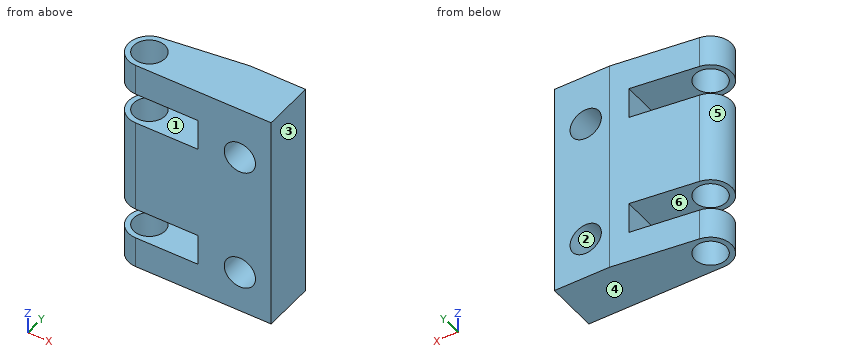
```python
from build123d import *

# Parameters (mm, degrees)
SKETCH_1_R          = 1.5
EXTRUDE_1_DEPTH     = 21
SKETCH_3_W          = 8
SKETCH_3_H          = 3
CUT_EXTRUDE_1_DEPTH = 6
SKETCH_4_R          = 1.5
CUT_EXTRUDE_2_DEPTH = 21


with BuildPart() as part:
    # 草图1 → 凸台-拉伸1 (new body)
    with BuildSketch(Plane.XY):
        with BuildLine():
            Line((-1.936190112, 5), (3.350194549, 5))
            Line((3.350194549, 5), (3.350194549, 0))
            Line((3.350194549, 0), (0, 0))
            Line((0, 0), (-9.649805451, 0))
            ThreePointArc((-9.649805451, 0), (-11.645783707, 1.873229335), (-9.902836943, 3.983929198))
            Line((-9.902836943, 3.983929198), (-1.936190112, 5))
        make_face()
        with Locations((-9.649805451, 2)):
            Circle(SKETCH_1_R, mode=Mode.SUBTRACT)
    extrude(amount=EXTRUDE_1_DEPTH)

    # 草图3 → 切除-拉伸1 (cut, through all)
    with BuildSketch(Plane(origin=(0, 0, 0), x_dir=(1, 0, 0), z_dir=(0, 1, 0))):
        with Locations((-7.649805451, -4.5)):
            Rectangle(SKETCH_3_W, SKETCH_3_H)
        with Locations((-7.649805451, -16.5)):
            Rectangle(SKETCH_3_W, SKETCH_3_H)
    extrude(amount=CUT_EXTRUDE_1_DEPTH, mode=Mode.SUBTRACT)

    # 草图4 → 切除-拉伸2 (cut)
    with BuildSketch(Plane(origin=(0, 5, 0), x_dir=(1, 0, 0), z_dir=(0, 1, 0))):
        with Locations((0.350194549, -4)):
            Circle(SKETCH_4_R)
        with Locations((0.350194549, -16)):
            Circle(SKETCH_4_R)
    extrude(amount=-CUT_EXTRUDE_2_DEPTH, mode=Mode.SUBTRACT)


solid = part.part
```
Input: part model. Units: mm. Frame: model coordinates. Face numbers are marked on the shaded views. A direction names the side the tool comes from. Give positions to 0.01 mm unless a question says otherwise; leave off trailing zeros. Order: outer loops, then holes, each group sorted by start corner. A loop starts at its lowest first (then second) coordinate and runs counter-clockwise, first axis right, second up.
1. Draft query along Z for the marked faces 1, 2, 3 and 4. Return one class per face: released by +Z, released by -Z, zero draft, split by the parting line, or undercut.
Computed:
face 1: undercut
face 2: undercut
face 3: zero draft
face 4: released by -Z
2. Cut plane A-A (y = 2). Return loops of the section in (x, z).
Computed:
outline: (-11.65, 0) - (-11.15, 0) - (-11.15, 3) - (-11.65, 3) - close; (-11.65, 6) - (-11.15, 6) - (-11.15, 15) - (-11.65, 15) - close; (-11.65, 18) - (-11.15, 18) - (-11.15, 21) - (-11.65, 21) - close; (-8.15, 0) - (3.35, 0) - (3.35, 21) - (-8.15, 21) - (-8.15, 18) - (-3.65, 18) - (-3.65, 15) - (-8.15, 15) - (-8.15, 6) - (-3.65, 6) - (-3.65, 3) - (-8.15, 3) - close; hole circle Ø3 at (0.35, 4); hole circle Ø3 at (0.35, 16)
3. Cut plane B-B (z = 16). Return loops of the section in (x, y).
Computed:
outline: (-3.65, 0) - (-1.15, 0) - (-1.15, 5) - (-1.94, 5) - (-3.65, 4.78) - close; (1.85, 0) - (3.35, 0) - (3.35, 5) - (1.85, 5) - close
4. Line query: probe 1 along Z at (x, y) = (-8, 2.2); probe 2 along X at (y, z) = (2.35, 14.75); probe 3 along X at (y, z) = (3.95, 4). Output: solid intervals per line, ascending.
Computed:
probe 1: z = 0 to 3, 6 to 15, 18 to 21
probe 2: x = -11.62 to -11.11, -8.19 to -0.48, 1.18 to 3.35
probe 3: x = -3.65 to -1.15, 1.85 to 3.35
5. Cut plane D-D (z = 9.5). Return loops of the section in (x, y).
Computed:
outline: (-9.9, 3.98) arc R2 ccw to (-9.65, 0) - (3.35, 0) - (3.35, 5) - (-1.94, 5) - close; hole circle Ø3 at (-9.65, 2)
6. Pin query (flat end, axial travel): pin 1 Ø1.4 at (x, y) = (-9.5, 2) entering from +Z; pin 2 Ø0.9 at (y, z) = (3, 16) entering from -X. Return the tip coordinate at first contact, or that it passes through.
Computed:
pin 1: passes through
pin 2: stops at x = -3.65
7. Cut plane C-C (x = 0.5). Return loops of the section in (y, z).
Computed:
outline: (0, 0) - (5, 0) - (5, 2.51) - (0, 2.51) - close; (0, 5.49) - (5, 5.49) - (5, 14.51) - (0, 14.51) - close; (0, 17.49) - (5, 17.49) - (5, 21) - (0, 21) - close
8. Set-up query: the marked faces 5 and 6. Return all of +Z, -Z, +X, -X, +Y, -Y with unobstructed straight access to the full face (end or side cutting, diameter ignored); none if empty.
Computed:
face 5: +Z, -Z, -X
face 6: -X, +Y, -Y
